```python
from build123d import *

# Parameters (mm, degrees)
F0_W            = 42
F0_H            = 42
F1_DEPTH        = 7
F2_R            = 12
F3_DEPTH        = 25
F5_DEPTH        = 25
F7_D            = 3.3
F7_DEPTH        = 13.5
F7_TIP          = 0.9914200214
F8_SIZE         = 3
F10_D           = 4.4
F10_CBORE_D     = 8.25
F10_CBORE_DEPTH = 4


with BuildPart() as f1:
    # F0 (on Front) → F1 (new body)
    with BuildSketch(Plane.XZ):
        with Locations((21, 21)):
            Rectangle(F0_W, F0_H)
    extrude(amount=F1_DEPTH)

    # F2 (on face) → F3 (cut)
    with BuildSketch(Plane.XZ.offset(7)):
        with Locations((21, 21)):
            Circle(F2_R)
    extrude(amount=-F3_DEPTH, mode=Mode.SUBTRACT)

    # F4 (on face) → F5 (cut)
    with BuildSketch(Plane.XZ.offset(7)):
        with BuildLine():
            Line((13.0627460668, 30), (0, 30))
            Line((0, 30), (0, 0))
            Line((0, 0), (30, 0))
            Line((30, 0), (27.1547311219, 10.698578505))
            ThreePointArc((27.1547311219, 10.698578505), (11.3082217924, 13.9240240832), (13.0627460668, 30))
        make_face()
        with BuildLine():
            Line((22.0215506852, 30), (13.0627460668, 30))
            ThreePointArc((13.0627460668, 30), (11.3082217924, 13.9240240832), (27.1547311219, 10.698578505))
            Line((27.1547311219, 10.698578505), (22.0215506852, 30))
        make_face()
    extrude(amount=-F5_DEPTH, mode=Mode.SUBTRACT)

    # F7
    with Locations(Plane.XZ.offset(7)):
        with Locations((5.5, 36.5), (36.5, 36.5), (36.5, 5.5)):
            Hole(F7_D / 2, depth=F7_DEPTH)
            with Locations((0, 0, -(F7_DEPTH + F7_TIP / 2))):  # 118° drill point
                Cone(0, F7_D / 2, F7_TIP, mode=Mode.SUBTRACT)

    # F8
    f8_edges = [f1.edges().sort_by_distance(p)[0] for p in [
        (0, -3.5, 42),
        (42, -3.5, 42),
        (42, -3.5, 0),
    ]]
    chamfer(f8_edges, length=F8_SIZE)

    # F10 (through all)
    with Locations(Plane.XZ.offset(7)):
        with Locations((17.7627056837, 37.4929197133)):
            CounterBoreHole(F10_D / 2, F10_CBORE_D / 2, F10_CBORE_DEPTH)


solid = f1.part
```
Build history of the part. All positions in model axes, mm. A direction names the side the tool comes from. Give positions to 0.01 mm unless a question says otherwise; leave off trailing zeros. Loops run counter-clockwise (first coordinate to the right, second up) from the corner with the lowest first, then second, coordinate; pieces in that order, holes last. Notation, with made-up numbers: (23.5, 5.25) -> (36.5, 5.25) arc R28 ccw to (36.5, 31.25) -> close; hole circle Ø8 at (-17.5, -32). An arc over 180 degrees is marked (long way). One line per question, with ' | ' between items.
Q1. Cut at A-A, the plane x = 36.5. Write the cut outline in (y, z), plus the area to 3 significant figures.
Filled sheet:
outline: (-7, 0) -> (0, 0) -> (0, 3.85) -> (-7, 3.85) -> close; (-7, 7.15) -> (0, 7.15) -> (0, 34.85) -> (-7, 34.85) -> close; (-7, 38.15) -> (0, 38.15) -> (0, 42) -> (-7, 42) -> close | area: 248 mm²
Q2. Cut at C-C, the plane y = -5.5. Write the cut outline in (x, z) (3 decimals).
Filled sheet:
outline: (0, 30) -> (13.063, 30) arc R12 cw (long way) to (27.155, 10.699) -> (30, 0) -> (39, 0) -> (42, 3) -> (42, 39) -> (39, 42) -> (3, 42) -> (0, 39) -> close; hole circle Ø3.3 at (5.5, 36.5); hole circle Ø8.25 at (17.763, 37.493); hole circle Ø3.3 at (36.5, 5.5); hole circle Ø3.3 at (36.5, 36.5)
Q3. Drop flat-ended pins along their axis: pin 1 (1 mm diameter, centred on x = 23, y = -5.5, fed in from -Z); pin 2 (2 mm diameter, centred on x = 9, y = -3.5, fed in from -Z); pin 3 (4 mm diameter, centred on x = 19.5, z = 36.5, fed in from -Y). Give the stop position or say it passes through.
Filled sheet:
pin 1: stops at z = 32.74 | pin 2: stops at z = 30 | pin 3: stops at y = -3
Q4. Pull direction Z, two halves, no side cores. Call faces 1 (the cylindrical face through (15.73, -1.48, 36.65)), 2 (the flat face through (30, -7, 31)), 3 (the flat face through (21, -3, 42)), 4 (the flat face through (40, -3, 1)): pulls with the +Z half, pulls with the -Z half, needs draft (parallel to the pull), parting line crosses it, or undercut.
Filled sheet:
face 1: undercut | face 2: needs draft | face 3: pulls with the +Z half | face 4: pulls with the -Z half
Q5. Cut at B-B, the plane z = 36.5. Write the cut outline in (x, y).
Filled sheet:
outline: (0, -7) -> (3.85, -7) -> (3.85, 0) -> (0, 0) -> close; (7.15, -7) -> (13.76, -7) -> (13.76, -3) -> (15.8, -3) -> (15.8, 0) -> (7.15, 0) -> close; (19.73, -3) -> (21.77, -3) -> (21.77, -7) -> (34.85, -7) -> (34.85, 0) -> (19.73, 0) -> close; (38.15, -7) -> (42, -7) -> (42, 0) -> (38.15, 0) -> close
Q6. Cut at D-D, the plane x = 17. Write the cut outline in (y, z).
Filled sheet:
outline: (-7, 32.31) -> (0, 32.31) -> (0, 35.43) -> (-3, 35.43) -> (-3, 33.44) -> (-7, 33.44) -> close; (-7, 41.55) -> (-3, 41.55) -> (-3, 39.56) -> (0, 39.56) -> (0, 42) -> (-7, 42) -> close
Q7. Drill centre lines: line 1 along Z through (x, y) = (35.5, -4); line 2 along X through (y, z) = (-4.75, 35.5); line 3 along Z through (x, y) = (5.5, -2.5). Where is each one in solid material? Low to high. Write a range as [from, to].
Filled sheet:
line 1: z = [0, 4.19], [6.81, 35.19], [37.81, 42] | line 2: x = [0, 4.19], [6.81, 14.15], [21.37, 35.19], [37.81, 42] | line 3: z = [30, 34.85], [38.15, 42]
Q8. Tool access for faces 5 (the cylindrical face through (37.716, -3.451, 37.615)), 6 (the flat face through (20, -3, 36)), 7 (the flat face through (7, -4, 30)): list every direction of +Z, -Z, +X, -X, +Y, -Y with a clear straight run to the whole face (end or side of a thin tool).
Filled sheet:
face 5: +Y, -Y | face 6: -Y | face 7: -Z, -X, +Y, -Y
